from build123d import *

# Parameters (mm, degrees)
F0_R     = 14.6685
F1_DEPTH = 25.4
F2_R     = 7.0993
F3_DEPTH = 34.29


with BuildPart() as f1:
    # F0 (on Front) → F1 (new body)
    with BuildSketch(Plane.XZ):
        with BuildLine():
            Line((-19.812, -72.4535), (0, -72.4535))
            Line((0, -72.4535), (19.812, -72.4535))
            Line((19.812, -72.4535), (27.146323, -20.0025))
            Line((27.146323, -20.0025), (26.9875, 0))
            ThreePointArc((26.9875, 0), (0, 26.9875), (-26.9875, 0))
            Line((-26.9875, 0), (-26.9875, -20.0025))
            Line((-26.9875, -20.0025), (-19.812, -72.4535))
        make_face()
        Circle(F0_R, mode=Mode.SUBTRACT)
    extrude(amount=F1_DEPTH)

    # F2 (on face) → F3 (cut)
    with BuildSketch(Plane(origin=(0, 0, -72.4535), x_dir=(1, 0, 0), z_dir=(0, 0, -1))):
        with Locations((0, 12.7)):
            Circle(F2_R)
    extrude(amount=-F3_DEPTH, mode=Mode.SUBTRACT)


solid = f1.part
Could you check a few things on this model? Use its own coordinates, in mm. A direction names the side the tool comes from. Coordinates: 2 decimals unless noted, no trailing zeros. Order: outer loops, then holes, each group sorted by start corner. A loop starts at its lowest first (then second) coordinate and runs counter-clockwise, first axis right, second up. Notation, with made-up numbers: (38.5, 11) -> (77.5, 11) arc R23 ccw to (77.5, 41) -> close; hole circle Ø1 at (31, -4). An arc over 180 degrees is marked (long way). One line per item, written item: value. Start each with the question number.
1) Imagine slicing it at B-B on z = -4. List the corners of the cut face in (x, y) for me, plus the area to 3 significant figures.
2) If I drill on L1, parallel to Y at x = 0, z = -64.5; L2, parallel to Z at x = 0, y = -20; L3, parallel to Z at x = 0, y = -19.25, over which ranges is the centre line in solid material (lowest first)? Write a range as [from, to].
3) Imagine slicing it at D-D on z = -60. List the corners of the cut face in (x, y) for me.
4) We'd pull the mould along X, two halves only. Please class faces 1 (the cylindrical face through (-10.811, -12.522, 9.914)), 2 (the flat face through (0, -25.4, -22)), 3 (the flat face through (-26.988, -13, -10)): +X half, -X half, draft (parallel to the pull), parting line (faces both ways), or undercut.
5) Which directions (+Z, -Z, +X, -X, +Y, -Y) give clear straight access to the entire face, cutting with the end or side of a thin tool? Please do faces 4 (the flat face through (0, -13, -38.164)), 5 (the flat face through (23.428, -12.522, -46.595)).
6) Imagine slicing it at A-A on x = 0. List the corners of the cut face in (y, z) for me.
7) Imagine slicing it at C-C on y = -12.7. List the corners of the cut face in (x, z) for me (1 decimal).
8) I'm going to push flat-ended pins straight in: pin 1 (2 mm diameter, centred on y = -7, z = -56.5, fed in from +X); pin 2 (4 mm diameter, centred on x = 17, y = -6, fed in from +Z); pin 3 (4.5 mm diameter, centred on x = 2, y = -12.5, fed in from -Z); pin 4 (6 mm diameter, centred on y = -20.5, z = -18.5, fed in from +X). Where does each tip first touch, or does it pass through?
Answer list:
1. outline: (-26.99, -25.4) -> (-14.11, -25.4) -> (-14.11, 0) -> (-26.99, 0) -> close; (14.11, -25.4) -> (27.02, -25.4) -> (27.02, 0) -> (14.11, 0) -> close
1. area: 655 mm2
2. L1: y = [-25.4, -19.8], [-5.6, 0]
2. L2: z = [-72.45, -14.67], [14.67, 26.99]
2. L3: z = [-38.16, -14.67], [14.67, 26.99]
3. outline: (-21.52, -25.4) -> (21.55, -25.4) -> (21.55, 0) -> (-21.52, 0) -> close; hole circle Ø14.2 at (0, -12.7)
4. face 1: undercut
4. face 2: draft
4. face 3: -X half
5. face 4: -Z
5. face 5: -Z, +X, +Y, -Y
6. outline: (-25.4, -72.45) -> (-19.8, -72.45) -> (-19.8, -38.16) -> (-5.6, -38.16) -> (-5.6, -72.45) -> (0, -72.45) -> (0, -14.67) -> (-25.4, -14.67) -> close; (-25.4, 14.67) -> (0, 14.67) -> (0, 26.99) -> (-25.4, 26.99) -> close
7. outline: (-27, -20) -> (-19.8, -72.5) -> (-7.1, -72.5) -> (-7.1, -38.2) -> (7.1, -38.2) -> (7.1, -72.5) -> (19.8, -72.5) -> (27.1, -20) -> (27, 0) arc R27 ccw to (-27, 0) -> close; hole circle Ø29.3 at (0, 0)
8. pin 1: stops at x = 22.18
8. pin 2: stops at z = 22.43
8. pin 3: stops at z = -38.16
8. pin 4: stops at x = 27.15
